from build123d import *

# Parameters (mm, degrees)
F0_R     = 30
F0_R_2   = 10.25
F1_DEPTH = 4
F2_DEPTH = 25
F3_R     = 3
F4_SIZE  = 2.99999
F6_SIZE2 = 0.7
F6_SIZE  = 0.2
F7_START = -6
F7_DEPTH = 19
F8_D     = 4.65
F8_DEPTH = 8
F8_TIP   = 1.3970009392
F9_R     = 2


# Not quite as in the source:
# - a fillet or chamfer is up to 0.001 mm smaller than in the source, because OpenCascade refuses the exact size


with BuildPart() as f1:
    # F0 (on Top) → F1 (new body)
    with BuildSketch(Plane.XY):
        Circle(F0_R)
        with BuildLine():
            ThreePointArc((8, 11.7924764151), (12.5909193469, 6.6731739075), (14.25, 0))
            ThreePointArc((14.25, 0), (-6.6731739075, -12.5909193469), (-8, 11.7924764151))
            Line((-8, 11.7924764151), (-8, 20.25))
            Line((-8, 20.25), (8, 20.25))
            Line((8, 20.25), (8, 11.7924764151))
        make_face(mode=Mode.SUBTRACT)
        with BuildLine():
            ThreePointArc((-8, 11.7924764151), (0, 14.25), (8, 11.7924764151))
            Line((8, 11.7924764151), (8, 20.25))
            Line((8, 20.25), (-8, 20.25))
            Line((-8, 20.25), (-8, 11.7924764151))
        make_face()
        with BuildLine():
            ThreePointArc((-8, 11.7924764151), (-6.6731739075, -12.5909193469), (14.25, 0))
            ThreePointArc((14.25, 0), (12.5909193469, 6.6731739075), (8, 11.7924764151))
            ThreePointArc((8, 11.7924764151), (0, 14.25), (-8, 11.7924764151))
        make_face()
        Circle(F0_R_2, mode=Mode.SUBTRACT)
    extrude(amount=F1_DEPTH)

    # F0 (on Top) → F2 (join)
    with BuildSketch(Plane.XY):
        with BuildLine():
            ThreePointArc((-8, 11.7924764151), (0, 14.25), (8, 11.7924764151))
            Line((8, 11.7924764151), (8, 20.25))
            Line((8, 20.25), (-8, 20.25))
            Line((-8, 20.25), (-8, 11.7924764151))
        make_face()
        with BuildLine():
            ThreePointArc((-8, 11.7924764151), (-6.6731739075, -12.5909193469), (14.25, 0))
            ThreePointArc((14.25, 0), (12.5909193469, 6.6731739075), (8, 11.7924764151))
            ThreePointArc((8, 11.7924764151), (0, 14.25), (-8, 11.7924764151))
        make_face()
        Circle(F0_R_2, mode=Mode.SUBTRACT)
    extrude(amount=F2_DEPTH)

    # F3
    f3_edges = [f1.edges().sort_by_distance(p)[0] for p in [
        (-8, 11.792476, 14.5),
        (8, 11.792476, 14.5),
        (8, 20.25, 14.5),
        (-8, 20.25, 14.5),
    ]]
    fillet(f3_edges, radius=F3_R)

    # F4 (size 3 in the source; OpenCascade refuses exactly that, so slightly less here)
    f4_edges = [f1.edges().sort_by_distance(p)[0] for p in [
        (0, -14.25, 4),
        (-8, 15.268841, 4),
        (8, 15.268841, 4),
    ]]
    chamfer(f4_edges, length=F4_SIZE)

    # F6
    f6_edges = [f1.edges().sort_by_distance(p)[0] for p in [
        (-10.25, 0, 0),
        (-30, 0, 0),
    ]]
    f6_side = f1.faces().sort_by_distance((-29.151472, 0, 0))[0]
    chamfer(f6_edges, length=F6_SIZE, length2=F6_SIZE2, reference=f6_side)

    # F5 (on face) → F7 (cut)
    with BuildSketch(Plane(origin=(0, 20.25, 0), x_dir=(-1, 0, 0), z_dir=(0, 1, 0)).offset(F7_START)):
        Polygon((-4.36, 18.5172471737), (-4.36, 13.4827528263), (0, 10.9655056527), (4.36, 13.4827528263), (4.36, 18.5172471737), (0, 21.0344943473), align=None)
    extrude(amount=-F7_DEPTH, mode=Mode.SUBTRACT)

    # F8
    with Locations(Plane(origin=(0, 20.25, 0), x_dir=(-1, 0, 0), z_dir=(0, 1, 0))):
        with Locations((0, 16)):
            Hole(F8_D / 2, depth=F8_DEPTH)
            with Locations((0, 0, -(F8_DEPTH + F8_TIP / 2))):  # 118° drill point
                Cone(0, F8_D / 2, F8_TIP, mode=Mode.SUBTRACT)

    # F9
    f9_edges = [f1.edges().sort_by_distance(p)[0] for p in [
        (-30, 0, 4),
        (0, -14.25, 25),
    ]]
    fillet(f9_edges, radius=F9_R)


solid = f1.part
Check sheet for the modelled part. Datum: model origin and axes. Units: mm. A direction names the side the tool comes from. Give positions to 0.01 mm unless a question says otherwise; leave off trailing zeros. Order: outer loops, then holes, each group sorted by start corner. A loop starts at its lowest first (then second) coordinate and runs counter-clockwise, first axis right, second up. Notation, with made-up numbers: (36.5, -19) - (76.5, -19) arc R23 cw to (76.5, -1) - close; hole circle Ø2 at (83, -36). An arc over 180 degrees is marked (long way). Answer as CSV lines item,"result".
1. Go/stop test with flat-tipped pins: P1, Ø12, axis at x = -23, z = 4, coming from the -Y side; P2, Ø9.5, axis at x = 1, z = 15, coming from the -Y side; P3, Ø6, axis at y = -7, z = 15.5, coming from the +X side. Record where each tip stops, or that it passes through.
Result sheet:
P1,"y = -24.52"
P2,"y = -14.25"
P3,"x = 13.68"
2. Mould release check, pull along X, two halves, no side actions. Record for faces 1 (the face through (-29.97, 1.32, 1.34)), 2 (the face through (2.21, 12.35, 12.24)), 3 (the face through (0, 20.25, 13)): released by +X, released by -X, zero draft, split by the parting line, or undercut.
Result sheet:
face 1,"split by the parting line"
face 2,"undercut"
face 3,"zero draft"
3. Section check D-D (z = 2.75). Record the boundary of the cut face in (x, y).
Result sheet:
outline,"circle Ø59.71 at (0, 0); hole circle Ø20.5 at (0, 0)"
4. Section check A-A (z = 16). Record the boundary of the cut face in (x, y) (3 decimals), then the cut area to 3 significant figures.
Result sheet:
outline,"(-9.087, 10.977) arc R14.25 ccw (long way) to (9.087, 10.977) arc R3 cw to (8, 13.288) - (8, 17.25) arc R3 ccw to (5, 20.25) - (2.325, 20.25) - (2.325, 14.25) - (4.36, 14.25) - (4.36, 9.276) arc R10.25 cw (long way) to (-4.36, 9.276) - (-4.36, 14.25) - (-2.325, 14.25) - (-2.325, 20.25) - (-5, 20.25) arc R3 ccw to (-8, 17.25) - (-8, 13.288) arc R3 cw to start"
area,"348 mm²"
5. Tool access check on faces 4 (the face through (7.43, 15.3, 24.4)), 5 (the face through (-8, 15, 15)), 6 (the face through (2, 14.25, 14)), 7 (the face through (-0.07, 19.68, 24.4)). Record the directions out of +Z, -Z, +X, -X, +Y, -Y that give a thin tool (end or side, any length) a straight path to the whole face; none if there is none.
Result sheet:
face 4,"+Z, +X, +Y"
face 5,"+Z, -X, +Y"
face 6,"none"
face 7,"+Z, +X, -X, +Y"
6. Section check C-C (x = 1). State how many separate pieces and enclosed holes the cut face has, then the cut area to 3 significant figures.
Result sheet:
separate pieces,"3"
enclosed holes,"0"
area,"398 mm²"
7. Section check B-B (z = 12). Record the boundary of the cut face in (x, y), then the cut area to 3 significant figures.
Result sheet:
outline,"(-9.09, 10.98) arc R14.25 ccw (long way) to (9.09, 10.98) arc R3 cw to (8, 13.29) - (8, 17.25) arc R3 ccw to (5, 20.25) - (-5, 20.25) arc R3 ccw to (-8, 17.25) - (-8, 13.29) arc R3 cw to start; hole (-1.79, 10.09) arc R10.25 ccw (long way) to (1.79, 10.09) - (1.79, 14.25) - (-1.79, 14.25) - close"
area,"399 mm²"
8. Scan lines: probe 1 along Z at (x, y) = (-23.5, 5); probe 2 along Y at (x, z) = (2.5, 18.5); probe 3 along X at (y, z) = (-9.5, 14.5). Record each from-to range of solid material in increasing order. Write a range as from..to.
Result sheet:
probe 1,"0..4"
probe 2,"-14.03..-9.94, 14.25..20.25"
probe 3,"-10.62..-3.85, 3.85..10.62"
